```python
from build123d import *

# Parameters (mm, degrees)
SKETCH1_W           = 12.34
SKETCH1_H           = 10.05
BOSS_EXTRUDE1_DEPTH = 11.09
SKETCH2_R           = 3.75
CUT_EXTRUDE1_DEPTH  = 5
SKETCH4_R           = 2.44
BOSS_EXTRUDE2_DEPTH = 5
SKETCH6_R           = 0.375
CUT_EXTRUDE2_DEPTH  = 8
SKETCH13_R          = 0.555
SKETCH13_W          = 1.23
SKETCH13_H          = 0.5
SKETCH13_W_2        = 0.5
SKETCH13_H_2        = 1.2
SKETCH13_W_3        = 1.03
SKETCH13_W_4        = 0.455661697
SKETCH13_W_5        = 0.46
SKETCH13_W_6        = 0.68
SKETCH13_H_3        = 0.37
BOSS_EXTRUDE3_DEPTH = 2.31
FILLET2_R           = 0.5
FILLET3_R           = 0.5
FILLET4_SIZE        = 0.5


with BuildPart() as part:
    # Sketch1 → Boss-Extrude1 (new body)
    with BuildSketch(Plane(origin=(0, 0, 0), x_dir=(1, 0, 0), z_dir=(0, 1, 0))):
        Rectangle(SKETCH1_W, SKETCH1_H)
    extrude(amount=BOSS_EXTRUDE1_DEPTH)

    # Sketch2 → Cut-Extrude1 (cut)
    with BuildSketch(Plane(origin=(6.17, 0, 0), x_dir=(0, 0, -1), z_dir=(1, 0, 0))):
        with Locations((0, 5.42)):
            Circle(SKETCH2_R)
    extrude(amount=-CUT_EXTRUDE1_DEPTH, mode=Mode.SUBTRACT)

    # Sketch4 → Boss-Extrude2 (add)
    with BuildSketch(Plane(origin=(1.17, 0, 0), x_dir=(0, 0, -1), z_dir=(1, 0, 0))):
        with Locations(Location((0, 5.42, 0), (0, 0, 180))):
            Circle(SKETCH4_R)
    extrude(amount=BOSS_EXTRUDE2_DEPTH)

    # Sketch6 → Cut-Extrude2 (cut)
    with BuildSketch(Plane(origin=(6.17, 0, 0), x_dir=(0, 0, -1), z_dir=(1, 0, 0))):
        with Locations((0, 5.42)):
            Circle(SKETCH6_R)
    extrude(amount=-CUT_EXTRUDE2_DEPTH, mode=Mode.SUBTRACT)

    # Sketch13 → Boss-Extrude3 (add)
    with BuildSketch(Plane.XZ):
        with Locations(Location((3.425, 1.73, 0), (0, 0, 90))):
            Circle(SKETCH13_R)
        with Locations(Location((3.425, -1.73, 0), (0, 0, 90))):
            Circle(SKETCH13_R)
        with Locations((3.415, 4.775)):
            Rectangle(SKETCH13_W, SKETCH13_H)
        with Locations((-5.87, -2.755)):
            Rectangle(SKETCH13_W_2, SKETCH13_H_2)
        with Locations((-2.855, 4.775)):
            Rectangle(SKETCH13_W_3, SKETCH13_H)
        with Locations((-5.87, 2.755)):
            Rectangle(SKETCH13_W_2, SKETCH13_H_2)
        with Locations((-3.042169152, 0)):
            Rectangle(SKETCH13_W_4, SKETCH13_H_2)
        with Locations((0.955661697, 0)):
            Rectangle(SKETCH13_W_5, SKETCH13_H_2)
        with Locations((-2.855, -4.775)):
            Rectangle(SKETCH13_W_3, SKETCH13_H)
        with Locations((3.415, -4.775)):
            Rectangle(SKETCH13_W, SKETCH13_H)
        with Locations((-5.83, 0)):
            Rectangle(SKETCH13_W_6, SKETCH13_H_3)
    extrude(amount=BOSS_EXTRUDE3_DEPTH)

    # Fillet2
    fillet2_edges = [part.edges().sort_by_distance(p)[0] for p in [
        (-2.34, -2.31, -4.775),
        (-3.37, -2.31, -4.775),
        (4.03, -2.31, -4.775),
        (2.8, -2.31, -4.775),
        (4.03, -2.31, 4.775),
        (2.8, -2.31, 4.775),
        (-3.37, -2.31, 4.775),
        (-2.34, -2.31, 4.775),
    ]]
    fillet(fillet2_edges, radius=FILLET2_R)

    # Fillet3
    fillet3_edges = [part.edges().sort_by_distance(p)[0] for p in [
        (0, 11.09, 5.025),
        (0, 11.09, -5.025),
    ]]
    fillet(fillet3_edges, radius=FILLET3_R)

    # Fillet4
    # a fillet whose section is not a circle: 0.5 mm, written as the material it takes off along each edge
    with BuildSketch(Plane(origin=(2.435661697, -2.31, -0.6), x_dir=(0, 1, 0), z_dir=(-1, 0, 0)), Plane(origin=(-0.524338303, -2.31, 0.6), x_dir=(0, 1, 0), z_dir=(1, 0, 0))) as fillet4_piece_1:
        with BuildLine():
            Bezier((FILLET4_SIZE, 0), (0, 0), (0, -FILLET4_SIZE), weights=[1, 0.035355339, 1])
            Line((0, -FILLET4_SIZE), (0, 0))
            Line((0, 0), (FILLET4_SIZE, 0))
        make_face()
    extrude(amount=2.96, mode=Mode.SUBTRACT)
    with BuildSketch(Plane(origin=(-1.564338303, -2.31, -0.6), x_dir=(0, 1, 0), z_dir=(-1, 0, 0)), Plane(origin=(-4.52, -2.31, 0.6), x_dir=(0, 1, 0), z_dir=(1, 0, 0))) as fillet4_piece_2:
        with BuildLine():
            Bezier((FILLET4_SIZE, 0), (0, 0), (0, -FILLET4_SIZE), weights=[1, 0.035355339, 1])
            Line((0, -FILLET4_SIZE), (0, 0))
            Line((0, 0), (FILLET4_SIZE, 0))
        make_face()
    extrude(amount=2.955661697, mode=Mode.SUBTRACT)
    with BuildSketch(Plane(origin=(-7.37, -2.31, -3.355), x_dir=(0, 1, 0), z_dir=(1, 0, 0)), Plane(origin=(-4.37, -2.31, -2.155), x_dir=(0, 1, 0), z_dir=(-1, 0, 0))) as fillet4_piece_3:
        with BuildLine():
            Bezier((FILLET4_SIZE, 0), (0, 0), (0, FILLET4_SIZE), weights=[1, 0.035355339, 1])
            Line((0, FILLET4_SIZE), (0, 0))
            Line((0, 0), (FILLET4_SIZE, 0))
        make_face()
    extrude(amount=3, mode=Mode.SUBTRACT)
    with BuildSketch(Plane(origin=(-4.37, -2.31, 2.155), x_dir=(0, 1, 0), z_dir=(-1, 0, 0)), Plane(origin=(-7.37, -2.31, 3.355), x_dir=(0, 1, 0), z_dir=(1, 0, 0))) as fillet4_piece_4:
        with BuildLine():
            Bezier((FILLET4_SIZE, 0), (0, 0), (0, -FILLET4_SIZE), weights=[1, 0.035355339, 1])
            Line((0, -FILLET4_SIZE), (0, 0))
            Line((0, 0), (FILLET4_SIZE, 0))
        make_face()
    extrude(amount=3, mode=Mode.SUBTRACT)


solid = part.part
```
Model file for the job. Use its own axes, mm. A direction names the side the tool comes from. Coordinates: 2 decimals unless noted, no trailing zeros. Loops run counter-clockwise (first coordinate to the right, second up) from the corner with the lowest first, then second, coordinate; pieces in that order, holes last. Notation, with made-up numbers: M 30.5,2 L 69.5,2 A15 ccw 69.5,15 Z; hole C 23,17 d9. An arc over 180 degrees is marked long. Use CSV: the item, a comma, the result in double quotes. Start each with the question number.
1. Tool access for faces 1 (the flat face through (-6.12, -1, 3)), 2 (the flat face through (3, -1, -4.525)), 3 (the flat face through (1.17, 3, -1)), 4 (the flat face through (1.186, -1, 0)), 5 (the cylindrical face through (2.96, -1.14, -1.43)): list every direction of +Z, -Z, +X, -X, +Y, -Y with a clear straight run to the whole face (end or side of a thin tool).
2. Band-saw the part on A-A, the plane x = 2. List the corners of the cut face in (y, z) (3 decimals), then the cut area to 3 significant figures.
3. Flat gauge pins, fed straight in: pin 1 (0.6 mm diameter, centred on y = -1.5, z = -5, fed in from +X); pin 2 (1 mm diameter, centred on y = -1.5, z = 3, fed in from +X); pin 3 (3 mm diameter, centred on x = -1, z = 2.5, fed in from -Y). Where does each tip first touch, or does it go through?
4. Two-plate mould, pull along Y, no slides. Class faces 6 (the flat face through (3.4, -2.31, 1.7)), 7 (the cylindrical face through (3.705, 9.138, 0.488)), 8 (the flat face through (-5.62, -1, -3)): pulls with the +Y half, pulls with the -Y half, needs draft (parallel to the pull), parting line crosses it, or undercut.
5. Band-saw the part on D-D, the plane y = 7.5. List the corners of the cut face in (x, z) (3 decimals).
6. Band-saw the part on C-C, the plane z = 1.73. List the corners of the cut face in (x, y), then the cut area to 3 significant figures.
7. Band-saw the part on B-B, the plane y = 5.42. List the corners of the cut face in (x, z) (3 decimals), then the cut area to 3 significant figures.
8. Probe probe 1 along Y at (x, z) = (3.45, 0) (3 decimals); probe 2 along Y at (x, z) = (0.5, 0) (3 decimals); probe 3 along Y at (x, z) = (5.25, 2). List the from-to ranges inside material, lowest first. Write a range as [from, to].
Entries:
1,face 1,"+Z, -X, -Y"
1,face 2,"+X, -X, -Y"
1,face 3,"+X"
1,face 4,"+Z, -Z, +X, -Y"
1,face 5,"-Y"
2,outline,"M 0,-5.025 L 10.59,-5.025 A0.5 ccw 11.09,-4.525 L 11.09,4.525 A0.5 ccw 10.59,5.025 L 0,5.025 Z; C 5.42,0 d4.88; hole C 5.42,0 d7.5; hole C 5.42,0 d0.75"
2,area,"85.4 mm2"
3,pin 1,"stops at x = 4.03"
3,pin 2,"stops at x = -5.62"
3,pin 3,"stops at y = 0"
4,face 6,"pulls with the -Y half"
4,face 7,"undercut"
4,face 8,"needs draft"
5,outline,"M -6.17,-5.025 L 6.17,-5.025 L 6.17,-3.12 L 1.17,-3.12 L 1.17,-1.276 L 6.17,-1.276 L 6.17,1.276 L 1.17,1.276 L 1.17,3.12 L 6.17,3.12 L 6.17,5.025 L -6.17,5.025 Z"
6,outline,"M -6.17,0 L 2.87,0 L 2.87,-2.31 L 3.98,-2.31 L 3.98,0 L 6.17,0 L 6.17,2.09 L 1.17,2.09 L 1.17,3.7 L 6.17,3.7 L 6.17,7.14 L 1.17,7.14 L 1.17,8.75 L 6.17,8.75 L 6.17,11.09 L -6.17,11.09 Z"
6,area,"123 mm2"
7,outline,"M -6.17,-5.025 L 6.17,-5.025 L 6.17,-3.75 L 1.17,-3.75 L 1.17,-2.44 L 6.17,-2.44 L 6.17,-0.375 L -1.83,-0.375 L -1.83,0.375 L 6.17,0.375 L 6.17,2.44 L 1.17,2.44 L 1.17,3.75 L 6.17,3.75 L 6.17,5.025 L -6.17,5.025 Z"
7,area,"105 mm2"
8,probe 1,"y = [0, 1.67], [2.98, 5.045], [5.795, 7.86], [9.17, 11.09]"
8,probe 2,"y = [0, 5.045], [5.795, 11.09]"
8,probe 3,"y = [0, 2.25], [4.02, 6.82], [8.59, 11.09]"
